Verification items for the finished model (mm, model axes). A direction names the side the tool comes from. Round coordinates to 2 decimals unless told otherwise and drop trailing zeros. Order: outer loops, then holes, each group sorted by start corner. A loop starts at its lowest first (then second) coordinate and runs counter-clockwise, first axis right, second up. Notation, with made-up numbers: M 84.5,72.25 L 111.5,72.25 A14 ccw 111.5,92.25 Z; hole C 33.25,56.25 d9. An arc over 180 degrees is marked long. Use one line per item in the form item = value. Start each with the question number.
Item 1: Go/stop test with flat-tipped pins: pin 1 Ø1.8 at (x, z) = (-25.5, 18) entering from +Y; pin 2 Ø3.5 at (x, z) = (7.5, 7.5) entering from +Y; pin 3 Ø3 at (x, z) = (-11, -11.5) entering from +Y; pin 4 Ø1.6 at (x, z) = (25.5, -18.5) entering from +Y. Record where each tip stops, or that it passes through.
Item 2: Tool access check on faces 1 (the flat face through (0, 0, 0)), 2 (the flat face through (26, 18, 2)), 3 (the flat face through (26.5, 10, 0)). Record the directions out of +Z, -Z, +X, -X, +Y, -Y that give a thin tool (end or side, any length) a straight path to the whole face; none if there is none.
Item 3: Cross-section at A-A on y = 6.75. Count the separate pieces of the cut face and the enclosed holes in it, then the cut area to 3 significant figures.
Item 4: Cross-section at D-D on x = -15. Enter the section's corners in (y, z).
Item 5: Cross-section at C-C on z = 15. Enter the section's corners in (x, y), then the cut area to 3 significant figures.
Item 6: Cross-section at B-B on x = 0.5. Enter the section's corners in (y, z).
Item 7: Release check for a two-part mould opening along X. For faces 4 (the flat face through (-2.3, 5, -3)), 5 (the flat face through (-27.5, 10, 0)), 6 (the flat face through (0, 10, 20)) record: +X half, -X half, draft (parallel to the pull), parting line (faces both ways), or undercut.
Item 8: Thickness scan on probe 1 along X at (y, z) = (6.75, -2); probe 2 along X at (y, z) = (19.05, 18); probe 3 along X at (y, z) = (4, 17). Record the ranges inside material, lowest first. Write a range as [from, to].
from build123d import *

# Parameters (mm, degrees)
SKETCH_1_W          = 55
SKETCH_1_H          = 40
EXTRUDE_1_DEPTH     = 20
SKETCH_2_R          = 1
CUT_EXTRUDE_2_DEPTH = 3
SHELL_START         = 1
SHELL_1_DEPTH       = 19
SHELL_1_2_DEPTH     = 15
CHAMFER_2_SIZE      = 1
SKETCH_8_W          = 3
SKETCH_8_H          = 3
CUT_EXTRUDE_5_DEPTH = 10
SKETCH_10_W         = 1.5
SKETCH_10_H         = 10
EXTRUDE_2_DEPTH     = 3
SKETCH_11_W         = 0.5
SKETCH_11_H         = 5
SKETCH_11_W_2       = 15
SKETCH_11_H_2       = 0.5
EXTRUDE_6_DEPTH     = 5
SKETCH_11_7_R       = 1.5
EXTRUDE_7_DEPTH     = 7
SKETCH_11_8_W       = 1
SKETCH_11_8_H       = 5
SKETCH_11_8_W_2     = 5
SKETCH_11_8_H_2     = 1
EXTRUDE_8_DEPTH     = 9
CUT_EXTRUDE_6_DEPTH = 10
FILLET_1_R          = 0.3


# Read off the part's stored shape, not the designer's step: 抽壳1
with BuildPart() as part:
    # 草图1 → 凸台-拉伸1 (new body)
    with BuildSketch(Plane(origin=(0, 0, 0), x_dir=(1, 0, 0), z_dir=(0, 1, 0))):
        Rectangle(SKETCH_1_W, SKETCH_1_H)
    extrude(amount=EXTRUDE_1_DEPTH)

    # 草图2 → 切除-拉伸2 (cut)
    with BuildSketch(Plane(origin=(0, 20, 0), x_dir=(1, 0, 0), z_dir=(0, 1, 0))):
        with Locations(Location((-25.5, -18, 0), (0, 0, 270))):
            Circle(SKETCH_2_R)
        with Locations(Location((25.5, 18, 0), (0, 0, 270))):
            Circle(SKETCH_2_R)
    extrude(amount=-CUT_EXTRUDE_2_DEPTH, mode=Mode.SUBTRACT)

    # 抽壳1 outline → 抽壳1 (cut)
    with BuildSketch(Plane(origin=(0, 0, 0), x_dir=(1, 0, 0), z_dir=(0, 1, 0)).offset(SHELL_START)):
        with BuildLine():
            ThreePointArc((26.5, 16.267949192), (24.085786438, 16.585786438), (23.767949192, 19))
            Line((23.767949192, 19), (-26.5, 19))
            Line((-26.5, 19), (-26.5, -16.267949192))
            ThreePointArc((-26.5, -16.267949192), (-24.085786438, -16.585786438), (-23.767949192, -19))
            Line((-23.767949192, -19), (26.5, -19))
            Line((26.5, -19), (26.5, 16.267949192))
        make_face()
    extrude(amount=SHELL_1_DEPTH, mode=Mode.SUBTRACT)

    # Shell 1 2 outline → Shell 1 2 (cut)
    with BuildSketch(Plane(origin=(0, 0, 0), x_dir=(1, 0, 0), z_dir=(0, 1, 0)).offset(SHELL_START)):
        with BuildLine():
            Line((26.5, 16.267949192), (26.5, 19))
            Line((26.5, 19), (23.767949192, 19))
            ThreePointArc((23.767949192, 19), (24.085786438, 16.585786438), (26.5, 16.267949192))
        make_face()
        with BuildLine():
            ThreePointArc((-23.767949192, -19), (-24.085786438, -16.585786438), (-26.5, -16.267949192))
            Line((-26.5, -16.267949192), (-26.5, -19))
            Line((-26.5, -19), (-23.767949192, -19))
        make_face()
    extrude(amount=SHELL_1_2_DEPTH, mode=Mode.SUBTRACT)

    # 倒角2
    chamfer_2_edges = [part.edges().sort_by_distance(p)[0] for p in [
        (0, 0, -20),
        (27.5, 0, 0),
        (0, 0, 20),
        (-27.5, 0, 0),
        (-27.5, 10, -20),
        (27.5, 10, -20),
        (27.5, 10, 20),
        (-27.5, 10, 20),
    ]]
    chamfer(chamfer_2_edges, length=CHAMFER_2_SIZE)

    # 草图8 → 切除-拉伸5 (cut)
    with BuildSketch(Plane(origin=(0, 0, -20), x_dir=(-1, 0, 0), z_dir=(0, 0, -1))):
        with Locations((0, 2.5)):
            Rectangle(SKETCH_8_W, SKETCH_8_H)
    extrude(amount=-CUT_EXTRUDE_5_DEPTH, mode=Mode.SUBTRACT)

    # 草图10 → 凸台-拉伸2 (add)
    with BuildSketch(Plane(origin=(0, 20, 0), x_dir=(1, 0, 0), z_dir=(0, 1, 0))):
        with Locations((25.75, -7)):
            Rectangle(SKETCH_10_W, SKETCH_10_H)
    extrude(amount=-EXTRUDE_2_DEPTH)

    # 草图11 → 凸台-拉伸6 (add)
    with BuildSketch(Plane(origin=(0, 1, 0), x_dir=(1, 0, 0), z_dir=(0, 1, 0))):
        with Locations((25.35, 3.45)):
            Rectangle(SKETCH_11_W, SKETCH_11_H)
        with Locations((12.1, 10.2)):
            Rectangle(SKETCH_11_W_2, SKETCH_11_H_2)
        with Locations((12.1, -3.3)):
            Rectangle(SKETCH_11_W_2, SKETCH_11_H_2)
        with Locations((-1.15, 3.45)):
            Rectangle(SKETCH_11_W, SKETCH_11_H)
    extrude(amount=EXTRUDE_6_DEPTH)

    # 草图11<7> → 凸台-拉伸7 (add)
    with BuildSketch(Plane(origin=(0, 1, 0), x_dir=(1, 0, 0), z_dir=(0, 1, 0))):
        with Locations(Location((4.7, 16.413896805, 0), (0, 0, 270))):
            Circle(SKETCH_11_7_R)
        with Locations(Location((11.7, 16.413896805, 0), (0, 0, 270))):
            Circle(SKETCH_11_7_R)
        with Locations(Location((18.7, 16.413896805, 0), (0, 0, 270))):
            Circle(SKETCH_11_7_R)
        with Locations(Location((17.1, -7.952490826, 0), (0, 0, 270))):
            Circle(SKETCH_11_7_R)
        with Locations(Location((7.1, -7.952490826, 0), (0, 0, 270))):
            Circle(SKETCH_11_7_R)
    extrude(amount=EXTRUDE_7_DEPTH)

    # 草图11<8> → 凸台-拉伸8 (add)
    with BuildSketch(Plane(origin=(0, 1, 0), x_dir=(1, 0, 0), z_dir=(0, 1, 0))):
        with Locations((-2.8, 3.45)):
            Rectangle(SKETCH_11_8_W, SKETCH_11_8_H)
        with Locations((12.1, -12.6)):
            Rectangle(SKETCH_11_8_W_2, SKETCH_11_8_H_2)
    extrude(amount=EXTRUDE_8_DEPTH)

    # 草图12 → 切除-拉伸6 (cut)
    with BuildSketch(Plane.XY.offset(12)):
        Polygon((26.3, 20), (25, 18.7), (25, 20), align=None)
    extrude(amount=-CUT_EXTRUDE_6_DEPTH, mode=Mode.SUBTRACT)

    # 圆角1
    fillet_1_edges = [part.edges().sort_by_distance(p)[0] for p in [
        (25, 18.7, 7),
        (25, 17, 7),
        (25, 17.85, 12),
        (25, 17.85, 2),
    ]]
    fillet(fillet_1_edges, radius=FILLET_1_R)


solid = part.part
Output values:
q1.pin_1 = 17
q1.pin_2 = 8
q1.pin_3 = 1
q1.pin_4 = 20
q2.face_1 = +Z, -Z, +X, -X, -Y
q2.face_2 = +Y
q2.face_3 = none
q3.separate_pieces = 8
q3.enclosed_holes = 1
q3.area = 229 mm2
q4.outline = M 0,-19 L 1,-20 L 20,-20 L 20,-19 L 1,-19 L 1,19 L 20,19 L 20,20 L 1,20 L 0,19 Z
q5.outline = M -27.5,1 L -26.5,0 L 26.5,0 L 27.5,1 L 27.5,20 L 26.5,20 L 26.5,1 L -26.5,1 L -26.5,20 L -27.5,20 Z
q5.area = 92.0 mm2
q6.outline = M 0,-19 L 1,-20 L 1,19 L 20,19 L 20,20 L 1,20 L 0,19 Z; M 4,-20 L 20,-20 L 20,-19 L 4,-19 Z
q7.face_4 = undercut
q7.face_5 = -X half
q7.face_6 = draft
q8.probe_1 = [-27.5, -26.5], [-3.3, -2.3], [26.5, 27.5]
q8.probe_2 = [-27.5, -26.5], [-24.5, -23.5], [26.5, 27.5]
q8.probe_3 = [-27.5, -26.5], [26.5, 27.5]
